Verification items for the finished model (mm, model axes). Face numbers are marked on the shaded views. A direction names the side the tool comes from. Coordinates: 2 decimals unless noted, no trailing zeros. Order: outer loops, then holes, each group sorted by start corner. A loop starts at its lowest first (then second) coordinate and runs counter-clockwise, first axis right, second up. Notation, with made-up numbers: (-6, 31) -> (30, 31) arc R18 ccw to (30, 66) -> close; hole circle Ø10 at (-38.5, 76). An arc over 180 degrees is marked (long way). Write item = value, one per line. Start each with the question number.
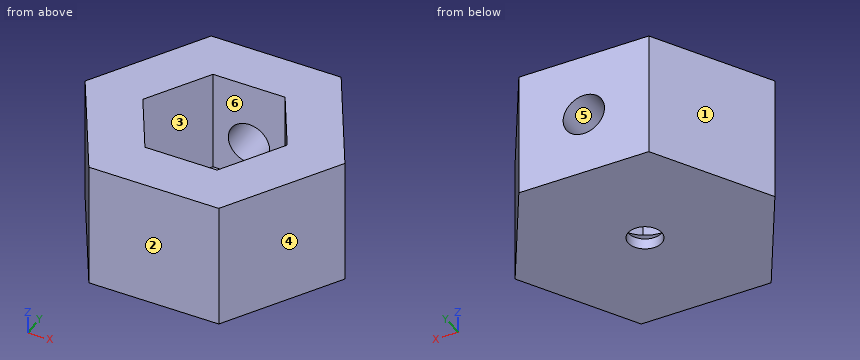
from build123d import *

# Parameters (mm, degrees)
BOSS_EXTRUDE1_DEPTH                            = 2.54
CSK_FOR_M3_FLAT_HEAD_MACHINE_SCREW1_AT_2_COUNT = 2
CSK_FOR_M3_FLAT_HEAD_MACHINE_SCREW1_AT_2_PITCH = 18.548356757
BOSS_EXTRUDE2_DEPTH                            = 12.7
M5X0_8_TAPPED_HOLE1_D                          = 4.2
M5X0_8_TAPPED_HOLE1_DEPTH                      = 5.08


with BuildPart() as part:
    # Sketch1 → Boss-Extrude1 (new body)
    # profile 1 of 2: a face of its own
    with BuildSketch(Plane.XY):
        Polygon((6.599113577, -11.43), (13.198227154, 0), (6.599113577, 11.43), (-6.599113577, 11.43), (-13.198227154, 0), (-6.599113577, -11.43), align=None)
        Polygon((-3.666174209, -6.35), (3.666174209, -6.35), (7.332348419, 0), (3.666174209, 6.35), (-3.666174209, 6.35), (-7.332348419, 0), align=None, mode=Mode.SUBTRACT)
    # profile 2 of 2: a face of its own
    with BuildSketch(Plane.XY):
        Polygon((-7.332348419, 0), (-3.666174209, -6.35), (3.666174209, -6.35), (7.332348419, 0), (3.666174209, 6.35), (-3.666174209, 6.35), align=None)
    extrude(amount=BOSS_EXTRUDE1_DEPTH)

    # Sketch3 → CSK for M3 Flat Head Machine Screw1 (revolve, cut)
    with BuildSketch(Plane(origin=(0, 0, 2.54), x_dir=(0, -1, 0), z_dir=(1, 0, 0))):
        Polygon((0, 0), (0, 2.54), (1.7, 2.54), (1.7, 1.45), (3.15, 0), align=None)
    csk_for_m3_flat_head_machine_screw1 = revolve(axis=Axis((0, 0, 8.89), (0, 0, -1)), mode=Mode.SUBTRACT)

    # CSK for M3 Flat Head Machine Screw1 at 2: CSK for M3 Flat Head Machine Screw1 ×2
    with Locations(*[Vector(-0.9274068813992224, 0.37405410883101997, 0) * (i * CSK_FOR_M3_FLAT_HEAD_MACHINE_SCREW1_AT_2_PITCH) for i in range(1, CSK_FOR_M3_FLAT_HEAD_MACHINE_SCREW1_AT_2_COUNT)]):
        add(csk_for_m3_flat_head_machine_screw1, mode=Mode.SUBTRACT)

    # Sketch1<4> → Boss-Extrude2 (add)
    with BuildSketch(Plane.XY):
        Polygon((6.599113577, 11.43), (-6.599113577, 11.43), (-13.198227154, 0), (-6.599113577, -11.43), (6.599113577, -11.43), (13.198227154, 0), align=None)
        Polygon((3.666174209, -6.35), (7.332348419, 0), (3.666174209, 6.35), (-3.666174209, 6.35), (-7.332348419, 0), (-3.666174209, -6.35), align=None, mode=Mode.SUBTRACT)
    extrude(amount=BOSS_EXTRUDE2_DEPTH)

    # M5x0.8 Tapped Hole1
    with Locations(Plane(origin=(0, 11.43, 0), x_dir=(1, 0, 0), z_dir=(0, 1, 0))):
        with Locations((0, -6.35)):
            Hole(M5X0_8_TAPPED_HOLE1_D / 2, depth=M5X0_8_TAPPED_HOLE1_DEPTH)


solid = part.part
Item 1: Section check A-A (x = 0). Record the boundary of the cut face in (y, z), then the cut area to 3 significant figures.
Item 2: Gauge pin test, flat ends, axial feed: P1, Ø4.5, axis at x = 0, y = 0, coming from the +Z side; P2, Ø1, axis at y = -2.5, z = 5.5, coming from the +X side; P3, Ø2, axis at x = -0.5, z = 7, coming from the +Y side. Record the tip position at first contact, or that the pin passes through.
Item 3: Mould release check, pull along X, two halves, no side actions. Record for the marked faces 1, 2 and 3: pulls with the +X half, pulls with the -X half, needs draft (parallel to the pull), parting line crosses it, or undercut.
Item 4: Section check D-D (y = 6.75). Record the boundary of the cut face in (x, z).
Item 5: Section check B-B (z = 11). Record the boundary of the cut face in (x, y).
Item 6: Tool access check on the marked faces 4, 5 and 6. Record the directions out of +Z, -Z, +X, -X, +Y, -Y that give a thin tool (end or side, any length) a straight path to the whole face; none if there is none.
Item 7: Section check C-C (z = 6.35). Record the boundary of the cut face in (x, y), then the cut area to 3 significant figures.
Item 8: Thickness scan on line 1 (Y direction, x = 0, z = 0.3); line 2 (Y direction, x = 0.25, z = 2.75); line 3 (Z direction, x = 4, y = 1). Record the ranges inside material, lowest first.
Filled sheet:
q1.outline = (-11.43, 0) -> (-1.7, 0) -> (-1.7, 1.09) -> (-3.15, 2.54) -> (-6.35, 2.54) -> (-6.35, 12.7) -> (-11.43, 12.7) -> close; (1.7, 0) -> (11.43, 0) -> (11.43, 4.25) -> (6.35, 4.25) -> (6.35, 2.54) -> (3.15, 2.54) -> (1.7, 1.09) -> close; (6.35, 8.45) -> (11.43, 8.45) -> (11.43, 12.7) -> (6.35, 12.7) -> close
q1.area = 129 mm^2
q2.P1 = 1.64
q2.P2 = 12.04
q2.P3 = -6.35
q3.face_1 = pulls with the -X half
q3.face_2 = needs draft
q3.face_3 = undercut
q4.outline = (-9.3, 0) -> (9.3, 0) -> (9.3, 12.7) -> (-9.3, 12.7) -> close; hole circle Ø4.2 at (0, 6.35)
q5.outline = (-13.2, 0) -> (-6.6, -11.43) -> (6.6, -11.43) -> (13.2, 0) -> (6.6, 11.43) -> (-6.6, 11.43) -> close; hole (-7.33, 0) -> (-3.67, -6.35) -> (3.67, -6.35) -> (7.33, 0) -> (3.67, 6.35) -> (-3.67, 6.35) -> close
q6.face_4 = +Z, -Z, +X, -Y
q6.face_5 = +Y
q6.face_6 = +Z
q7.outline = (-13.2, 0) -> (-6.6, -11.43) -> (6.6, -11.43) -> (13.2, 0) -> (6.6, 11.43) -> (2.1, 11.43) -> (2.1, 6.35) -> (3.67, 6.35) -> (7.33, 0) -> (3.67, -6.35) -> (-3.67, -6.35) -> (-7.33, 0) -> (-3.67, 6.35) -> (-2.1, 6.35) -> (-2.1, 11.43) -> (-6.6, 11.43) -> close
q7.area = 292 mm^2
q8.line_1 = -11.43 to -1.7, 1.7 to 11.43
q8.line_2 = -11.43 to -6.35, 6.35 to 11.43
q8.line_3 = 0 to 2.54
